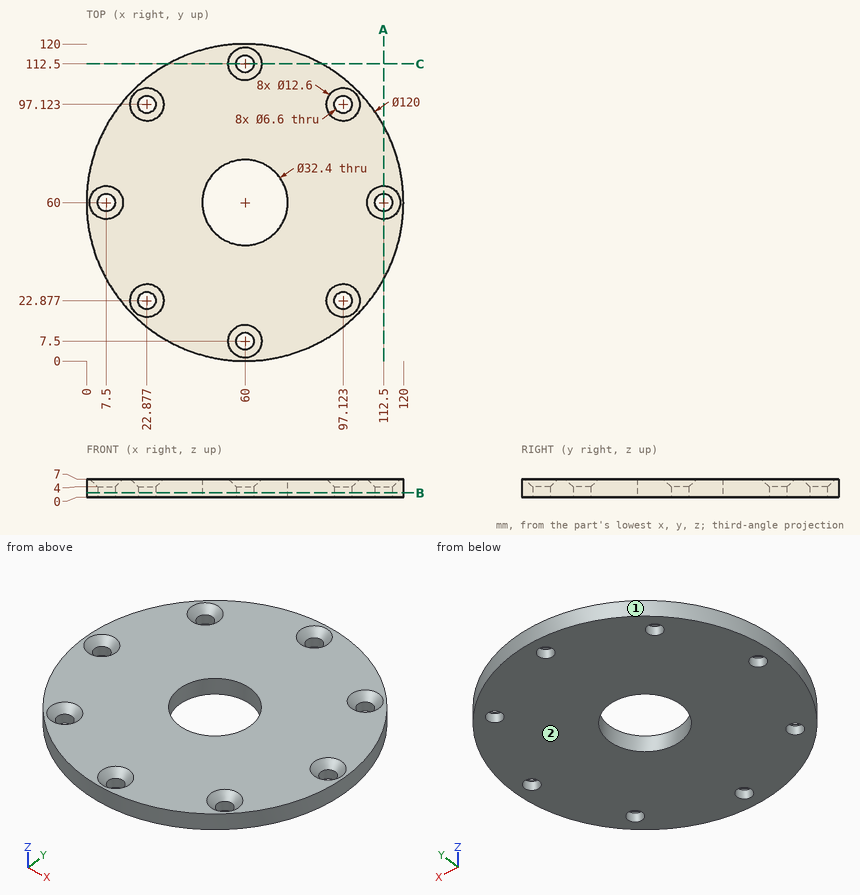
Verification items for this drawing (mm, ordinates from the low corner). Coordinates: 2 decimals unless noted, no trailing zeros. Order: outer loops, then holes, each group sorted by start corner. A loop starts at its lowest first (then second) coordinate and runs counter-clockwise, first axis right, second up. Notation, with made-up numbers: (89, 53) - (145, 53) arc R19 ccw to (145, 75) - close; hole circle Ø8 at (88.5, 10). An arc over 180 degrees is marked (long way). Answer in a Markdown table with one row per item. Add a question column.
1. Section check B-B (z = 1.75). Give the number of separate pieces and of enclosed holes in the cut face, plus the area to 3 significant figures.
2. Draft check along Y on the marked faces 1 and 2. Enter one of: +Y half, -Y half, draft (parallel to the pull), parting line (faces both ways), or undercut.
3. Material ranges on L1, parallel to Y at x = 60, z = 2.8; L2, parallel to X at y = 95, z = 2.25; L3, parallel to X at y = 27, z = 5.75, recorded low to high. Write a range as [from, to].
4. Gauge pin test, flat ends, axial feed: pin 1 Ø4 at (x, z) = (106.5, 5.5) entering from -Y; pin 2 Ø4 at (x, y) = (97.12, 22.88) entering from -Z; pin 3 Ø4 at (x, y) = (24.5, 45.5) entering from -Z; pin 4 Ø2 at (y, z) = (107, 4) entering from +X. Record the tip position at first contact, or that the pin passes through.
5. Section check A-A (x = 112.5). Enter the section's corners in (y, z), plus the area to 3 significant figures.
Data:
| question | item | result |
|---|---|---|
| 1 | separate pieces | 1 |
| 1 | enclosed holes | 9 |
| 1 | area | 10,200 mm² |
| 2 | face 1 | parting line |
| 2 | face 2 | draft |
| 3 | L1 | y = [0, 4.2], [10.8, 43.8], [76.2, 109.2], [115.8, 120] |
| 3 | L2 | x = [11.27, 20.35], [25.4, 94.6], [99.65, 108.73] |
| 3 | L3 | x = [9.89, 19.96], [25.79, 94.21], [100.04, 110.11] |
| 4 | pin 1 | stops at y = 19.75 |
| 4 | pin 2 | passes through |
| 4 | pin 3 | stops at z = 0 |
| 4 | pin 4 | stops at x = 98.52 |
| 5 | outline | (30.95, 0) - (56.7, 0) - (56.7, 4) - (53.7, 7) - (30.95, 7) - close; (63.3, 0) - (89.05, 0) - (89.05, 7) - (66.3, 7) - (63.3, 4) - close |
| 5 | area | 351 mm² |
